```python
from build123d import *

# Parameters (mm, degrees)
RESSALTO_EXTRUS_O1_DEPTH   = 20
CASCA1_T                   = -2
RESSALTO_EXTRUS_O2_DEPTH   = 10
FILETE1_R                  = 4
ESBO_O5_W                  = 23.985697769
ESBO_O5_H                  = 6
CORTE_EXTRUS_O1_DEPTH      = 15
ESBO_O6_W                  = 24.497787774
ESBO_O6_H                  = 6.032330751
CORTE_EXTRUS_O2_DEPTH      = 15
CORTE_EXTRUS_O3_DEPTH      = 15
CORTE_EXTRUS_O3_DEPTH_BACK = 15
ESBO_O7_W                  = 38.492647719
ESBO_O7_H                  = 2.75587166
ESBO_O7_H_2                = 3.088916175
ESBO_O7_H_3                = 3.326525112
ESBO_O7_W_2                = 34.690904734


with BuildPart() as part:
    # Esboço1 → Ressalto-extrusão1 (new body)
    with BuildSketch(Plane.XY):
        with BuildLine():
            Line((-35, 32.5), (35, 32.5))
            ThreePointArc((35, 32.5), (42.071067812, 29.571067812), (45, 22.5))
            Line((45, 22.5), (45, -22.5))
            ThreePointArc((45, -22.5), (42.071067812, -29.571067812), (35, -32.5))
            Line((35, -32.5), (-35, -32.5))
            ThreePointArc((-35, -32.5), (-42.071067812, -29.571067812), (-45, -22.5))
            Line((-45, -22.5), (-45, 22.5))
            ThreePointArc((-45, 22.5), (-42.071067812, 29.571067812), (-35, 32.5))
        make_face()
    extrude(amount=RESSALTO_EXTRUS_O1_DEPTH)

    # Casca1
    casca1_openings = [part.faces().sort_by_distance(p)[0] for p in [
        (0, 0, 20),
    ]]
    offset(amount=CASCA1_T, openings=casca1_openings, kind=Kind.INTERSECTION)

    # Esboço2 → Ressalto-extrusão2 (add)
    with BuildSketch(Plane(origin=(0, 0, 0), x_dir=(-1, 0, 0), z_dir=(0, 0, -1))):
        with BuildLine():
            Line((-30.08601431, 32.5), (-15.268763233, 32.5))
            Line((-15.268763233, 32.5), (-15.268763233, 10.675395158))
            Line((-15.268763233, 10.675395158), (-30.08601431, 10.675395158))
            ThreePointArc((-30.08601431, 10.675395158), (-37.157082122, 13.604327346), (-40.08601431, 20.675395158))
            Line((-40.08601431, 20.675395158), (-40.08601431, 22.5))
            ThreePointArc((-40.08601431, 22.5), (-37.157082122, 29.571067812), (-30.08601431, 32.5))
        make_face()
        with BuildLine():
            Line((14.243643453, 32.5), (29.06089453, 32.5))
            ThreePointArc((29.06089453, 32.5), (36.131962342, 29.571067812), (39.06089453, 22.5))
            Line((39.06089453, 22.5), (39.06089453, 20.675395158))
            ThreePointArc((39.06089453, 20.675395158), (36.131962342, 13.604327346), (29.06089453, 10.675395158))
            Line((29.06089453, 10.675395158), (14.243643453, 10.675395158))
            Line((14.243643453, 10.675395158), (14.243643453, 32.5))
        make_face()
    extrude(amount=RESSALTO_EXTRUS_O2_DEPTH)

    # Filete1
    filete1_edges = [part.edges().sort_by_distance(p)[0] for p in [
        (-21.652268991, 10.675395158, -10),
        (-36.131962342, 13.604327346, -10),
        (-39.06089453, 21.587697579, -10),
        (-36.131962342, 29.571067812, -10),
        (22.677388772, 10.675395158, -10),
        (37.157082122, 13.604327346, -10),
        (40.08601431, 21.587697579, -10),
        (37.157082122, 29.571067812, -10),
        (-21.652268991, 32.5, -10),
        (22.677388772, 32.5, -10),
    ]]
    fillet(filete1_edges, radius=FILETE1_R)

    # Esboço5 → Corte-extrusão1 (cut)
    with BuildSketch(Plane(origin=(0, 10.675395158, 0), x_dir=(-1, 0, 0), z_dir=(0, -1, 0))):
        with Locations((-24.546243996, 3)):
            Rectangle(ESBO_O5_W, ESBO_O5_H)
    extrude(amount=-CORTE_EXTRUS_O1_DEPTH, mode=Mode.SUBTRACT)

    # Esboço6 → Corte-extrusão2 (cut)
    with BuildSketch(Plane.XZ.offset(-10.675395158)):
        with Locations((-22.916938832, -3.016165375)):
            Rectangle(ESBO_O6_W, ESBO_O6_H)
    extrude(amount=-CORTE_EXTRUS_O2_DEPTH, mode=Mode.SUBTRACT)

    # Esboço7 → Corte-extrusão3 (cut, two sides: drawn at the far end of the back side and taken through both)
    with BuildSketch(Plane(origin=(0, 0, 0), x_dir=(-1, 0, 0), z_dir=(0, 0, -1)).offset(-CORTE_EXTRUS_O3_DEPTH_BACK)):
        with Locations((-45.552020228, -1.37793583)):
            Rectangle(ESBO_O7_W, ESBO_O7_H)
        with Locations((-45.552020228, -8.577290605)):
            Rectangle(ESBO_O7_W, ESBO_O7_H_2)
        with Locations((-45.552020228, -17.250016789)):
            Rectangle(ESBO_O7_W, ESBO_O7_H_3)
        with Locations((46.165029276, -1.37793583)):
            Rectangle(ESBO_O7_W_2, ESBO_O7_H)
        with Locations((46.165029276, -8.577290605)):
            Rectangle(ESBO_O7_W_2, ESBO_O7_H_2)
        with Locations((46.165029276, -17.250016789)):
            Rectangle(ESBO_O7_W_2, ESBO_O7_H_3)
    extrude(amount=CORTE_EXTRUS_O3_DEPTH + CORTE_EXTRUS_O3_DEPTH_BACK, mode=Mode.SUBTRACT)


solid = part.part
```
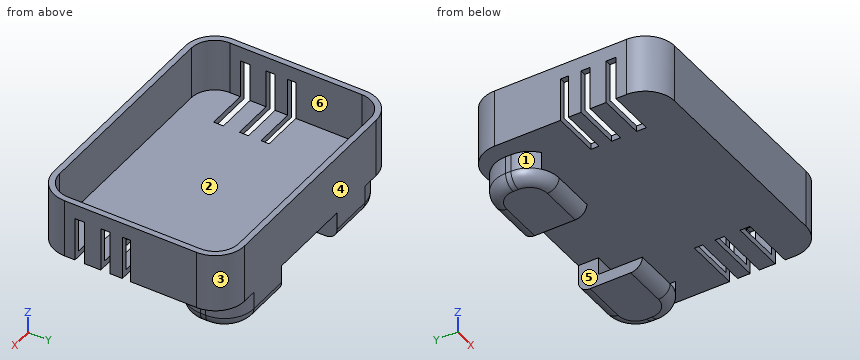
Check sheet for the modelled part. Datum: model origin and axes. Units: mm. Face numbers are marked on the shaded views. A direction names the side the tool comes from. Coordinates: 2 decimals unless noted, no trailing zeros. Loops run counter-clockwise (first coordinate to the right, second up) from the corner with the lowest first, then second, coordinate; pieces in that order, holes last.
1) Sectioned sample at A-A (z = 18). Record the boundary of the cut face in (x, y), and give its area (3 significant figures).
2) Material ranges on probe 1 along X at (y, z) = (7, 15.5); probe 2 along Y at (x, z) = (-12, 6); probe 3 along Y at (x, z) = (-39, 0.5), recorded low to high.
3) Access from +Z, -Z, +X, -X, +Y, -Y to the whole of each face (thin tool, end or side, straight path). Record for the marked faces 1, 2 and 3.
4) Release check for a two-part mould opening along Y. For the marked faces 4, 5 and 6 record: released by +Y, released by -Y, zero draft, split by the parting line, or undercut.
5) Sectioned sample at C-C (x = -10.5). Record the boundary of the cut face in (y, z), and give its area (3 significant figures).
6) Gauge pin test, flat ends, axial feed: pin 1 (1.8 mm diameter, centred on x = -19.5, z = -1.5, fed in from -Y); pin 2 (0.6 mm diameter, centred on y = -18, z = 0.5, fed in from -X); pin 3 (1 mm diameter, centred on x = 44, y = -2, fed in from -Z); pin 4 (6 mm diameter, centred on y = -11, z = -3.5, fed in from -X). Record the tip position at first contact, or that the pin passes through.
7) Sectioned sample at D-D (z = -4). Record the boundary of the cut face in (x, y), and give its area (3 significant figures).
8) Sectioned sample at B-B (y = -8). Record the boundary of the cut face in (x, z), and give its area (3 significant figures).
Check sheet entries:
1. outline: (-45, -22.5) arc R10 ccw to (-35, -32.5) - (35, -32.5) arc R10 ccw to (45, -22.5) - (45, 22.5) arc R10 ccw to (35, 32.5) - (-35, 32.5) arc R10 ccw to (-45, 22.5) - close; hole (-43, -22.5) arc R8 ccw to (-35, -30.5) - (35, -30.5) arc R8 ccw to (43, -22.5) - (43, 22.5) arc R8 ccw to (35, 30.5) - (-35, 30.5) arc R8 ccw to (-43, 22.5) - close
1. area: 573 mm2
2. probe 1: x = -45 to -43, 43 to 45
2. probe 2: y = -32.5 to -30.5, 30.5 to 32.5
2. probe 3: y = -31.67 to -18.91, -15.59 to -10.12, -7.03 to -2.76, 0 to 31.67
3. face 1: -Z, -X, -Y
3. face 2: +Z
3. face 3: +Z, -Z, +X, +Y
4. face 4: released by +Y
4. face 5: zero draft
4. face 6: undercut
5. outline: (-32.5, 0) - (32.5, 0) - (32.5, 20) - (30.5, 20) - (30.5, 2) - (-30.5, 2) - (-30.5, 20) - (-32.5, 20) - close
5. area: 202 mm2
6. pin 1: stops at y = 25.68
6. pin 2: stops at x = -28.82
6. pin 3: stops at z = 15
6. pin 4: passes through
7. outline: (-39.06, 20.68) arc R10 ccw to (-35.17, 12.76) - (-35.17, 25.68) - (-14.24, 25.68) - (-14.24, 32.5) - (-29.06, 32.5) arc R10 ccw to (-39.06, 22.5) - close; (15.27, 25.68) - (36.54, 25.68) - (36.54, 13.04) arc R10 ccw to (40.09, 20.68) - (40.09, 22.5) arc R10 ccw to (30.09, 32.5) - (15.27, 32.5) - close
7. area: 373 mm2
8. outline: (-45, 15) - (-43, 15) - (-43, 20) - (-45, 20) - close; (-28.82, 0) - (26.31, 0) - (26.31, 2) - (-28.82, 2) - close; (43, 15) - (45, 15) - (45, 20) - (43, 20) - close
8. area: 130 mm2
